```python
from build123d import *

# Parameters (mm, degrees)
F0_R          = 6.349014
F1_DEPTH      = 1.27
F2_DEPTH      = 1.27
F3_W          = 52.788634
F3_H          = 5.319013
F4_DEPTH      = 1.27
F5_R          = 6.442503
F6_DEPTH      = 1.27
F8_DEPTH      = 12.7
F8_DEPTH_BACK = 25.4
F10_DEPTH     = 12.7


with BuildPart() as f1:
    # F0 (on Top) → F1 (new body)
    with BuildSketch(Plane.XY):
        with Locations((-57.772908, 15.168429)):
            Circle(F0_R)
    extrude(amount=F1_DEPTH)

    # F0 (on Top) → F2 (join)
    with BuildSketch(Plane.XY):
        with Locations((-57.772908, 15.168429)):
            Circle(F0_R)
    extrude(amount=F2_DEPTH)

    # F3 (on Top) → F4 (join)
    with BuildSketch(Plane.XY):
        with Locations((-26.394317, 15.146691)):
            Rectangle(F3_W, F3_H)
    extrude(amount=F4_DEPTH)

    # F5 (on Top) → F6 (join)
    with BuildSketch(Plane.XY):
        with Locations((6.190753, 15.51234)):
            Circle(F5_R)
    extrude(amount=F6_DEPTH)

    # F7 (on face) → F8 (cut, two sides)
    with BuildSketch(Plane.XY.offset(1.27)) as f8_sk:
        Polygon((-54.338023, 13.185297), (-54.338023, 17.151561), (-57.772908, 19.134693), (-61.207794, 17.151561), (-61.207794, 13.185297), (-57.772908, 11.202165), align=None)
    extrude(amount=-F8_DEPTH, mode=Mode.SUBTRACT)
    extrude(f8_sk.sketch, amount=-F8_DEPTH_BACK, mode=Mode.SUBTRACT)

    # F9 (on face) → F10 (cut)
    with BuildSketch(Plane.XY.offset(1.27)):
        with BuildLine():
            Line((3.883671, 12.134312), (11.676623, 12.134312))
            ThreePointArc((11.676623, 12.134312), (15.03445, 15.492139), (11.676623, 18.849965))
            Line((11.676623, 18.849965), (3.883671, 18.849965))
            ThreePointArc((3.883671, 18.849965), (3.584843, 15.492139), (3.883671, 12.134312))
        make_face()
    extrude(amount=-F10_DEPTH, mode=Mode.SUBTRACT)


solid = f1.part
```
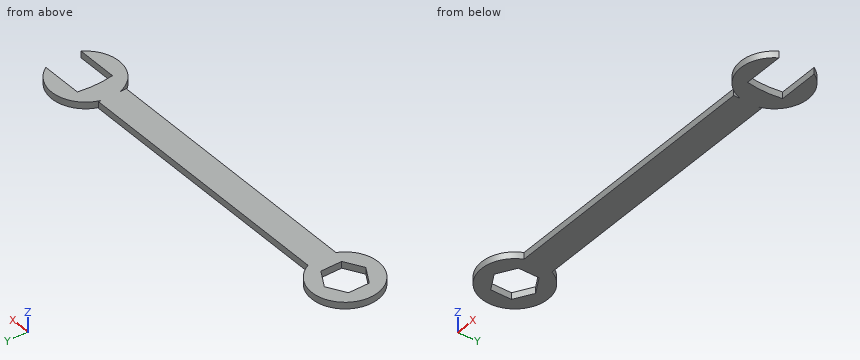
The listing builds one solid part. Answer for the finished solid, in the listing's coordinates (mm). Round coordinates to 2 decimals unless told otherwise and drop trailing zeros. Loops run counter-clockwise (first coordinate to the right, second up) from the corner with the lowest first, then second, coordinate; pieces in that order, holes last.
Q1. Section B-B, the plane y = 16 is taken. Determine the outline of the cut face in (x, z), then the cut area to 3 significant figures.
Q2. Section D-D, the plane y = 10.25 is taken. Determine the outline of the cut face in (x, z).
Q3. Section C-C, the plane x = -31 is taken. Determine the outline of the cut face in (y, z), then the cut area to 3 significant figures.
Q4. Given pin 1 Ø0.6 at (x, z) = (-17.5, 0.5) entering from +Y; pin 2 Ø0.6 at (y, z) = (15, 0.5) entering from +X; pin 3 Ø0.6 at (y, z) = (17.5, 1) entering from +X, each flat-ended and moving along its own axis, determine where each tip first touches the part or whether it passes through.
Q5. Find the intervals of material crossed by line 1 (X direction, y = 17.75, z = 0.3); line 2 (X direction, y = 15.5, z = 1.1); line 3 (X direction, y = 12.75, z = 0.5), in increasing order.
Completed:
1. outline: (-64.07, 0) - (-61.21, 0) - (-61.21, 1.27) - (-64.07, 1.27) - close; (-54.34, 0) - (3.59, 0) - (3.59, 1.27) - (-54.34, 1.27) - close
1. area: 77.2 mm2
2. outline: (-61.79, 0) - (-53.76, 0) - (-53.76, 1.27) - (-61.79, 1.27) - close; (2.47, 0) - (9.91, 0) - (9.91, 1.27) - (2.47, 1.27) - close
3. outline: (12.49, 0) - (17.81, 0) - (17.81, 1.27) - (12.49, 1.27) - close
3. area: 6.76 mm2
4. pin 1: stops at y = 17.81
4. pin 2: stops at x = 3.6
4. pin 3: stops at x = 3.73
5. line 1: x = -63.57 to -60.17, -55.37 to 0, 0.15 to 3.72
5. line 2: x = -64.11 to -61.21, -54.34 to 3.58
5. line 3: x = -63.64 to -60.45, -55.09 to 0, 0.37 to 3.78
